```python
from build123d import *

# Parameters (mm, degrees)
F1_DEPTH = 12.25
F2_W     = 2.44
F2_H     = 7.69
F3_DEPTH = 0.5
F6_DEPTH = 0.5
F7_R     = 0.5
F8_R     = 2.15
F8_R_2   = 2.05
F9_DEPTH = 0.501


with BuildPart() as f1:
    # F0 (on Front) → F1 (new body)
    with BuildSketch(Plane.XZ):
        Polygon((-12.885, 0.5), (-12.885, 0), (12.885, 0), (37.155871, 11.92), (39.595871, 11.92), (39.595871, 12.42), (37.155871, 12.42), (12.885, 0.5), align=None)
    extrude(amount=-F1_DEPTH)

    # F2 (on Top) → F3 (join)
    with BuildSketch(Plane.XY):
        with Locations((-14.105, 6.125)):
            Rectangle(F2_W, F2_H)
    extrude(amount=F3_DEPTH)

    # F5 (on offset) → F6 (join)
    with BuildSketch(Plane.YZ.offset(-15.325)):
        Polygon((2.28, 0.5), (9.97, 0.5), (9.97, 15.7), (8.64, 15.7), (7.258645, 15.7), (5.978645, 15.7), (4.678645, 15.7), (3.61, 15.7), (2.28, 15.7), align=None)
        Polygon((8.05, 11.42), (8.05, 1.5), (4.2, 1.5), (4.2, 11.42), (4.72, 11.42), (4.72, 12.8), (7.53, 12.8), (7.53, 11.42), align=None, mode=Mode.SUBTRACT)
        Polygon((8.64, 15.7), (9.97, 15.7), (9.97, 16), (8.97, 16), align=None)
        Polygon((7.258645, 15.7), (8.64, 15.7), (8.33, 16), (7.69, 16), align=None)
        Polygon((5.978645, 15.7), (7.258645, 15.7), (7.05, 16), (6.41, 16), align=None)
        Polygon((5.13, 16), (4.678645, 15.7), (5.978645, 15.7), (5.77, 16), align=None)
        Polygon((3.85, 16), (3.61, 15.7), (4.678645, 15.7), (4.49, 16), align=None)
        Polygon((2.28, 16), (2.28, 15.7), (3.61, 15.7), (3.28, 16), align=None)
    extrude(amount=F6_DEPTH)

    # F7
    f7_edges = [f1.edges().sort_by_distance(p)[0] for p in [
        (-14.825, 6.125, 0.5),
        (-15.325, 6.125, 0),
    ]]
    fillet(f7_edges, radius=F7_R)

    # F8 (on face) → F9 (cut, through all)
    with BuildSketch(Plane.XY.offset(0.5)):
        with Locations((-7.425, 6.125)):
            Circle(F8_R)
        with Locations((5.485, 6.125)):
            Circle(F8_R_2)
    extrude(amount=-F9_DEPTH, mode=Mode.SUBTRACT)


solid = f1.part
```
Design review of the part built by this model. Coordinates are the model's own, in mm. A direction names the side the tool comes from. Give positions to 0.01 mm unless a question says otherwise; leave off trailing zeros. Loops run counter-clockwise (first coordinate to the right, second up) from the corner with the lowest first, then second, coordinate; pieces in that order, holes last. Notation, with made-up numbers: (-1.5, 61.5) -> (55.5, 61.5) arc R33 ccw to (55.5, 100.5) -> close; hole circle Ø8 at (22, 62.5). An arc over 180 degrees is marked (long way). One line per item, written item: value.
Q1. We need section C-C on z = 8.5. Give the boundary of the cut face in (x, y) (3 decimals).
Numbers:
outline: (-15.325, 2.28) -> (-14.825, 2.28) -> (-14.825, 4.2) -> (-15.325, 4.2) -> close; (-15.325, 8.05) -> (-14.825, 8.05) -> (-14.825, 9.97) -> (-15.325, 9.97) -> close; (29.174, 0) -> (30.192, 0) -> (30.192, 12.25) -> (29.174, 12.25) -> close
Q2. Draft analysis for pull direction X (two halves, no side actions). For faces 1 (the flat face through (-15.325, 4, 8)), 2 (the flat face through (-15, 9.97, 7)), 3 (the flat face through (-1, 6, 0.5)), state which applies: pulls with the +X half, pulls with the -X half, needs draft (parallel to the pull), parting line crosses it, or undercut.
Numbers:
face 1: pulls with the -X half
face 2: needs draft
face 3: undercut
Q3. We need section A-A on x = -8. Give the boundary of the cut face in (y, z), and give its area (3 significant figures).
Numbers:
outline: (0, 0) -> (4.05, 0) -> (4.05, 0.5) -> (0, 0.5) -> close; (8.2, 0) -> (12.25, 0) -> (12.25, 0.5) -> (8.2, 0.5) -> close
area: 4.05 mm^2
Q4. We need section D-D on x = 26.5. Give the boundary of the cut face in (y, z).
Numbers:
outline: (0, 6.69) -> (12.25, 6.69) -> (12.25, 7.19) -> (0, 7.19) -> close
Q5. For L1, parallel to Z at x = 3.5, y = 4.5; L2, parallel to X at y = 9.75, z = 5 (3 decimals); L3, parallel to X at y = 6.5, z = 2.5, list the stretches that pass through material, from the lowest coordinate up.
Numbers:
L1: z = 0 to 0.5
L2: x = -15.325 to -14.825, 22.048 to 23.066
L3: x = 16.96 to 17.98
Q6. For pin 1 Ø2.5 at (x, z) = (-14, 6.5) entering from +Y; pin 2 Ø2.5 at (x, y) = (38, 5.5) entering from -Z; pin 3 Ø7 at (x, y) = (-7.425, 6.125) entering from +Z; pin 4 Ø0.6 at (x, y) = (-15, 8) entering from -Z, all flat-tipped, find the tip position at first contact; note any pin that passes through.
Numbers:
pin 1: stops at y = 9.97
pin 2: stops at z = 11.72
pin 3: stops at z = 0.5
pin 4: stops at z = 0
Q7. Machinability: for faces 4 (the flat face through (-15, 2.28, 7)), 5 (the flat face through (38, 6, 12.42)), 6 (the flat face through (38, 6, 11.92)), 7 (the flat face through (25.19, 6.039, 6.543)), which of the approach directions +Z, -Z, +X, -X, +Y, -Y give a long, thin tool a straight path to every point of the face, cutting with its end or side? Answer none if there is none.
Numbers:
face 4: +Z, -Z, -X, -Y
face 5: +Z, +X, +Y, -Y
face 6: -Z, +X, +Y, -Y
face 7: +Z, +Y, -Y
Q8. We need section B-B on y = 10.5. Give the boundary of the cut face in (x, z) (3 decimals).
Numbers:
outline: (-12.885, 0) -> (12.885, 0) -> (37.156, 11.92) -> (39.596, 11.92) -> (39.596, 12.42) -> (37.156, 12.42) -> (12.885, 0.5) -> (-12.885, 0.5) -> close
